Here's the drawing with two shaded views (mm, measured from the low corner). I have some questions. A direction names the side the tool comes from. Round coordinates to 2 decimals unless told otherwise and drop trailing zeros. Loops run counter-clockwise (first coordinate to the right, second up) from the corner with the lowest first, then second, coordinate; pieces in that order, holes last. Notation, with made-up numbers: (22, 59) -> (59, 59) arc R29 cw to (59, 79) -> close; hole circle Ø11 at (66.25, 42). An arc over 180 degrees is marked (long way). Write each question's results on one line, items separated by ' | '.
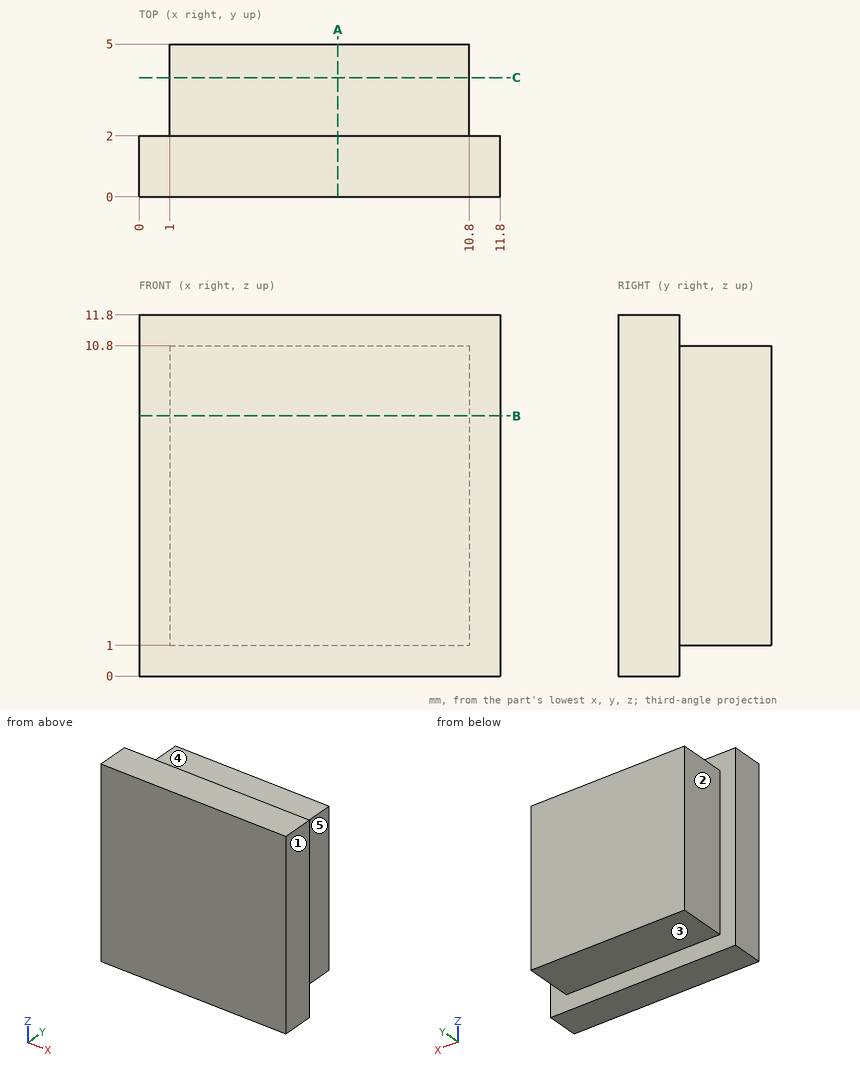
1. If we section it at B-B (z = 8.5): List the corners of the cut face in (x, y) for me, then the cut area to 3 significant figures.
Final values:
outline: (0, 0) -> (11.8, 0) -> (11.8, 2) -> (10.8, 2) -> (10.8, 5) -> (1, 5) -> (1, 2) -> (0, 2) -> close | area: 53.0 mm2
2. If we section it at A-A (x = 6.5): List the corners of the cut face in (y, z) for me.
Final values:
outline: (0, 0) -> (2, 0) -> (2, 1) -> (5, 1) -> (5, 10.8) -> (2, 10.8) -> (2, 11.8) -> (0, 11.8) -> close
3. Will these pins go through, and if not, where does the flat tip stop? pin 1 (1.5 mm diameter, centred on x = 5.5, y = 3, fed in from -Z); pin 2 (0.9 mm diameter, centred on y = 4, z = 4.5, fed in from +X); pin 3 (0.9 mm diameter, centred on y = 4, z = 4, fed in from -X).
Final values:
pin 1: z = 1 | pin 2: x = 10.8 | pin 3: x = 1
4. Please list where these lines run through material, in increasing order: line 1 (X direction, y = 3.2, z = 3.5); line 2 (Y direction, x = 11, z = 8). Write a range as from..to.
Final values:
line 1: 1..10.8 | line 2: 0..2
5. If we section it at C-C (y = 3.9): List the corners of the cut face in (x, z) for me, then the cut area to 3 significant figures.
Final values:
outline: (1, 1) -> (10.8, 1) -> (10.8, 10.8) -> (1, 10.8) -> close | area: 96.0 mm2
6. On a 3-axis mill with a long thin cutter (end or side, diameter ignored), from which of +Z, -Z, +X, -X, +Y, -Y can I reach the whole of each face in a straight line? I mean the marked faces 1, 2, 3, 4 and 5. Say none if no direction works.
Final values:
face 1: +Z, -Z, +X, +Y, -Y | face 2: +Z, -Z, -X, +Y | face 3: -Z, +X, -X, +Y | face 4: +Z, +X, -X, +Y | face 5: +Z, -Z, +X, +Y
